Build history of the part. All positions in model axes, mm. A direction names the side the tool comes from. Round coordinates to 2 decimals unless told otherwise and drop trailing zeros. Write each loop counter-clockwise with the first axis right and the second up, starting at its lowest first coordinate (ties: lowest second). Pieces come first, ordered by that corner, then holes. Notation, with made-up numbers: (33.5, 49) -> (51.5, 49) arc R24 cw to (51.5, 83) -> close; hole circle Ø11 at (-34.5, 41). An arc over 180 degrees is marked (long way). Answer in a Markdown table with one row per item.
```python
from build123d import *

# Parameters (mm, degrees)
SKETCH1_R           = 1.79
SKETCH1_R_2         = 12
BOSS_EXTRUDE1_DEPTH = 61.5
CUT_EXTRUDE1_DEPTH  = 29.5
CUT_EXTRUDE2_START  = -54.5
SKETCH3_R           = 3.79
CUT_EXTRUDE2_DEPTH  = 54.5
SKETCH4_OUTSIDE_W   = 108.324
SKETCH4_OUTSIDE_H   = 85.824
CUT_EXTRUDE3_DEPTH  = 28
CUT_EXTRUDE4_REACH  = 105.842
SKETCH5_R           = 1.65


with BuildPart() as part:
    # Sketch1 → Boss-Extrude1 (new body)
    with BuildSketch(Plane.XY):
        with BuildLine():
            Line((-5, 56.25), (-2.51, 56.25))
            ThreePointArc((-2.51, 56.25), (-2.156446609, 56.396446609), (-2.01, 56.75))
            Line((-2.01, 56.75), (-2.01, 60.75))
            ThreePointArc((-2.01, 60.75), (-1.863553391, 61.103553391), (-1.51, 61.25))
            Line((-1.51, 61.25), (3.5, 61.25))
            ThreePointArc((3.5, 61.25), (3.853553391, 61.103553391), (4, 60.75))
            Line((4, 60.75), (4, 60.054296555))
            ThreePointArc((4, 60.054296555), (7.537351062, 54.268735971), (14.299295775, 54.780270425))
            ThreePointArc((14.299295775, 54.780270425), (31.25, 60.25), (48.200704225, 54.780270425))
            ThreePointArc((48.200704225, 54.780270425), (54.962648938, 54.268735971), (58.5, 60.054296555))
            Line((58.5, 60.054296555), (58.5, 60.75))
            ThreePointArc((58.5, 60.75), (58.646446609, 61.103553391), (59, 61.25))
            Line((59, 61.25), (67.5, 61.25))
            ThreePointArc((67.5, 61.25), (72.5, 56.25), (67.5, 51.25))
            Line((67.5, 51.25), (65.01, 51.25))
            ThreePointArc((65.01, 51.25), (64.656446609, 51.103553391), (64.51, 50.75))
            Line((64.51, 50.75), (64.51, 41.751676566))
            ThreePointArc((64.51, 41.751676566), (64.656446609, 41.398123176), (65.01, 41.251676566))
            Line((65.01, 41.251676566), (67.5, 41.251676566))
            ThreePointArc((67.5, 41.251676566), (72.5, 36.251676566), (67.5, 31.251676566))
            Line((67.5, 31.251676566), (66.554952113, 31.258700852))
            ThreePointArc((66.554952113, 31.258700852), (62.117679705, 29.664703454), (59.697881988, 25.6181255))
            ThreePointArc((59.697881988, 25.6181255), (41.886466439, 4.271015925), (14.299295775, 7.719729575))
            ThreePointArc((14.299295775, 7.719729575), (7.537351062, 8.231264029), (4, 2.445703445))
            Line((4, 2.445703445), (4, 1.75))
            ThreePointArc((4, 1.75), (3.853553391, 1.396446609), (3.5, 1.25))
            Line((3.5, 1.25), (-1.51, 1.25))
            ThreePointArc((-1.51, 1.25), (-1.863553391, 1.396446609), (-2.01, 1.75))
            Line((-2.01, 1.75), (-2.01, 5.75))
            ThreePointArc((-2.01, 5.75), (-2.156446609, 6.103553391), (-2.51, 6.25))
            Line((-2.51, 6.25), (-5, 6.25))
            ThreePointArc((-5, 6.25), (-10, 11.25), (-5, 16.25))
            Line((-5, 16.25), (-2.51, 16.25))
            ThreePointArc((-2.51, 16.25), (-2.156446609, 16.396446609), (-2.01, 16.75))
            Line((-2.01, 16.75), (-2.01, 20.25))
            ThreePointArc((-2.01, 20.25), (-1.863553391, 20.603553391), (-1.51, 20.75))
            Line((-1.51, 20.75), (0, 20.75))
            Line((0, 20.75), (0, 41.75))
            Line((0, 41.75), (-1.51, 41.75))
            ThreePointArc((-1.51, 41.75), (-1.863553391, 41.896446609), (-2.01, 42.25))
            Line((-2.01, 42.25), (-2.01, 45.75))
            ThreePointArc((-2.01, 45.75), (-2.156446609, 46.103553391), (-2.51, 46.25))
            Line((-2.51, 46.25), (-5, 46.25))
            ThreePointArc((-5, 46.25), (-10, 51.25), (-5, 56.25))
        make_face()
        with Locations((-5, 51.25)):
            Circle(SKETCH1_R, mode=Mode.SUBTRACT)
        with Locations((-5, 11.25)):
            Circle(SKETCH1_R, mode=Mode.SUBTRACT)
        with Locations((67.5, 36.251676566)):
            Circle(SKETCH1_R, mode=Mode.SUBTRACT)
        with Locations((31.25, 31.25)):
            Circle(SKETCH1_R_2, mode=Mode.SUBTRACT)
        with Locations((67.5, 56.25)):
            Circle(SKETCH1_R, mode=Mode.SUBTRACT)
    extrude(amount=BOSS_EXTRUDE1_DEPTH)

    # Sketch2 → Cut-Extrude1 (cut)
    with BuildSketch(Plane.XY):
        with BuildLine():
            Line((0, 1.75), (0, 20.25))
            ThreePointArc((0, 20.25), (-0.146446609, 20.603553391), (-0.5, 20.75))
            Line((-0.5, 20.75), (0, 20.75))
            Line((0, 20.75), (0, 41.75))
            Line((0, 41.75), (-0.5, 41.75))
            ThreePointArc((-0.5, 41.75), (-0.146446609, 41.896446609), (0, 42.25))
            Line((0, 42.25), (0, 60.75))
            ThreePointArc((0, 60.75), (-0.146446609, 61.103553391), (-0.5, 61.25))
            Line((-0.5, 61.25), (0, 61.25))
            Line((0, 61.25), (62.5, 61.25))
            Line((62.5, 61.25), (63, 61.25))
            ThreePointArc((63, 61.25), (62.646446609, 61.103553391), (62.5, 60.75))
            Line((62.5, 60.75), (62.5, 31.758700852))
            ThreePointArc((62.5, 31.758700852), (62.646446609, 31.405147461), (63, 31.258700852))
            Line((63, 31.258700852), (66.554952113, 31.258700852))
            ThreePointArc((66.554952113, 31.258700852), (64.426142906, 30.924061927), (62.5, 29.957736232))
            Line((62.5, 29.957736232), (62.5, 1.25))
            Line((62.5, 1.25), (0, 1.25))
            Line((0, 1.25), (-0.5, 1.25))
            ThreePointArc((-0.5, 1.25), (-0.146446609, 1.396446609), (0, 1.75))
        make_face()
    extrude(amount=CUT_EXTRUDE1_DEPTH, mode=Mode.SUBTRACT)

    # Sketch3 → Cut-Extrude2 (cut)
    with BuildSketch(Plane.XY.offset(61.5).offset(CUT_EXTRUDE2_START)):
        with Locations((67.5, 36.251676566)):
            Circle(SKETCH3_R)
        with Locations((-5, 11.25)):
            Circle(SKETCH3_R)
        with Locations((-5, 51.25)):
            Circle(SKETCH3_R)
        with Locations((67.5, 56.25)):
            Circle(SKETCH3_R)
        with BuildLine():
            Line((64.51, 31.310229119), (64.51, 30.950386606))
            ThreePointArc((64.51, 30.950386606), (64.344469158, 30.897304147), (64.180307475, 30.840127679))
            ThreePointArc((64.180307475, 30.840127679), (64.419361538, 31.023134829), (64.51, 31.310229119))
        make_face()
    extrude(amount=CUT_EXTRUDE2_DEPTH, mode=Mode.SUBTRACT)

    # Sketch4 outside → Cut-Extrude3 (cut)
    with BuildSketch(Plane.XY.offset(61.5)):
        with Locations((31.25, 31.25)):
            Rectangle(SKETCH4_OUTSIDE_W, SKETCH4_OUTSIDE_H)
        Polygon((19.25, 43.02), (6.74, 43.02), (6.74, 19.48), (19.25, 19.48), (19.25, 23.5), (8.75, 23.5), (8.75, 39), (19.25, 39), align=None, mode=Mode.SUBTRACT)
        Polygon((43.25, 19.48), (55.76, 19.48), (55.76, 43.02), (43.25, 43.02), (43.25, 39), (53.75, 39), (53.75, 23.5), (43.25, 23.5), align=None, mode=Mode.SUBTRACT)
    extrude(amount=-CUT_EXTRUDE3_DEPTH, mode=Mode.SUBTRACT)

    # Cut-Extrude4: up to this face of the body (flat: up to its plane)
    cut_extrude4_end = Plane(part.part.faces().sort_by_distance((12.995, 19.48, 47.5))[0])
    # Sketch5 → Cut-Extrude4 (cut, up to the picked face)
    with BuildSketch(Plane(origin=(0, 43.02, 0), x_dir=(1, 0, 0), z_dir=(0, 1, 0)), mode=Mode.PRIVATE) as cut_extrude4_sk1:
        with Locations(Location((48.25, -58, 0), (0, 0, 270))):
            Circle(SKETCH5_R)
    cut_extrude4_tool1 = split(extrude(cut_extrude4_sk1.sketch, amount=-CUT_EXTRUDE4_REACH, mode=Mode.PRIVATE), bisect_by=cut_extrude4_end, keep=Keep.BOTH, mode=Mode.PRIVATE)
    # Sketch5 → Cut-Extrude4 (cut, up to the picked face)
    with BuildSketch(Plane(origin=(0, 43.02, 0), x_dir=(1, 0, 0), z_dir=(0, 1, 0)), mode=Mode.PRIVATE) as cut_extrude4_sk2:
        with Locations(Location((14.25, -58, 0), (0, 0, 270))):
            Circle(SKETCH5_R)
    cut_extrude4_tool2 = split(extrude(cut_extrude4_sk2.sketch, amount=-CUT_EXTRUDE4_REACH, mode=Mode.PRIVATE), bisect_by=cut_extrude4_end, keep=Keep.BOTH, mode=Mode.PRIVATE)
    add(cut_extrude4_tool1.solids().sort_by(Axis((48.25, 43.02, 58), (0, -1, 0)))[0], mode=Mode.SUBTRACT)
    add(cut_extrude4_tool2.solids().sort_by(Axis((14.25, 43.02, 58), (0, -1, 0)))[0], mode=Mode.SUBTRACT)


solid = part.part
```
Q1. Two-plate mould, pull along Y, no slides. Class faces 1 (the cylindrical face through (69.207, 56.788, 3.451)), 2 (the cylindrical face through (7.449, 54.315, 31.472)), 3 (the flat face through (-3, 11, 0)), 4 (the flat face through (65, 31.259, 15)): released by +Y, released by -Y, zero draft, split by the parting line, or undercut.
A:
| item | result |
|---|---|
| face 1 | undercut |
| face 2 | released by +Y |
| face 3 | zero draft |
| face 4 | released by -Y |
Q2. Drop flat-ended pins along their axis: P1, Ø0.7, axis at x = 66, z = 18, coming from the -Y side; P2, Ø10, axis at x = 5, y = 41.5, coming from the -Z side; P3, Ø1, axis at y = 20.5, z = 48.5, coming from the +X side. Give the stop position or say it passes through.
A:
| item | result |
|---|---|
| P1 | y = 31.26 |
| P2 | z = 29.5 |
| P3 | x = 55.76 |
Q3. Saw through at A-A on z = 58. State how many separate pieces and enclosed holes the cut face has, plus the area to 3 significant figures.
A:
| item | result |
|---|---|
| separate pieces | 6 |
| enclosed holes | 0 |
| area | 210 mm² |
Q4. Saw through at C-C on y = 11.25. Write the cut outline in (x, z).
A:
| item | result |
|---|---|
| outline | (-10, 0) -> (-6.79, 0) -> (-6.79, 7) -> (-8.79, 7) -> (-8.79, 33.5) -> (-10, 33.5) -> close; (-3.21, 0) -> (0, 0) -> (0, 29.5) -> (52.25, 29.5) -> (52.25, 33.5) -> (-1.21, 33.5) -> (-1.21, 7) -> (-3.21, 7) -> close |
Q5. Which spindle directions (+Z, -Z, +X, -X, +Y, -Y) get a long thin tool onto all of the face, cutting with end or side? Do faces 5 (the flat face through (-2.01, 59, 17)), 6 (the flat face through (0, 51, 15)), 7 (the flat face through (49, 19.48, 48)), 8 (the flat face through (66, 41.252, 17)). Say none if no direction does.
A:
| item | result |
|---|---|
| face 5 | +Z, -Z, -X, +Y |
| face 6 | -Z, +Y, -Y |
| face 7 | +Z, +X, -X, -Y |
| face 8 | +Z, -Z, +X |
Q6. Wall check: line 1 (Y direction, x = -5, z = 26.5); line 2 (Y direction, x = -5, z = 2); line 3 (Y direction, x = 13, z = 44). Give the ranges that are in metal, low to high. Write a range as [from, to].
A:
| item | result |
|---|---|
| line 1 | [6.25, 7.46], [15.04, 16.25], [46.25, 47.46], [55.04, 56.25] |
| line 2 | [6.25, 9.46], [13.04, 16.25], [46.25, 49.46], [53.04, 56.25] |
| line 3 | [19.48, 23.5], [39, 43.02] |
Q7. Saw through at B-B on x = 31.25. Write the cut outline in (y, z), plus the area to 3 significant figures.
A:
| item | result |
|---|---|
| outline | (2.25, 29.5) -> (19.25, 29.5) -> (19.25, 33.5) -> (2.25, 33.5) -> close; (43.25, 29.5) -> (60.25, 29.5) -> (60.25, 33.5) -> (43.25, 33.5) -> close |
| area | 136 mm² |
